The drawing under review shows one solid part. Ordinate dimensions are in mm from its lowest x, y, z. A direction names the side the tool comes from. Coordinates: 2 decimals unless noted, no trailing zeros. Order: outer loops, then holes, each group sorted by start corner. A loop starts at its lowest first (then second) coordinate and runs counter-clockwise, first axis right, second up. Notation, with made-up numbers: (80, 74) -> (102, 74) arc R19 ccw to (102, 86) -> close; hole circle Ø10 at (-21.5, 77.5). An arc over 180 degrees is marked (long way). Put each result on its own line as item: value.
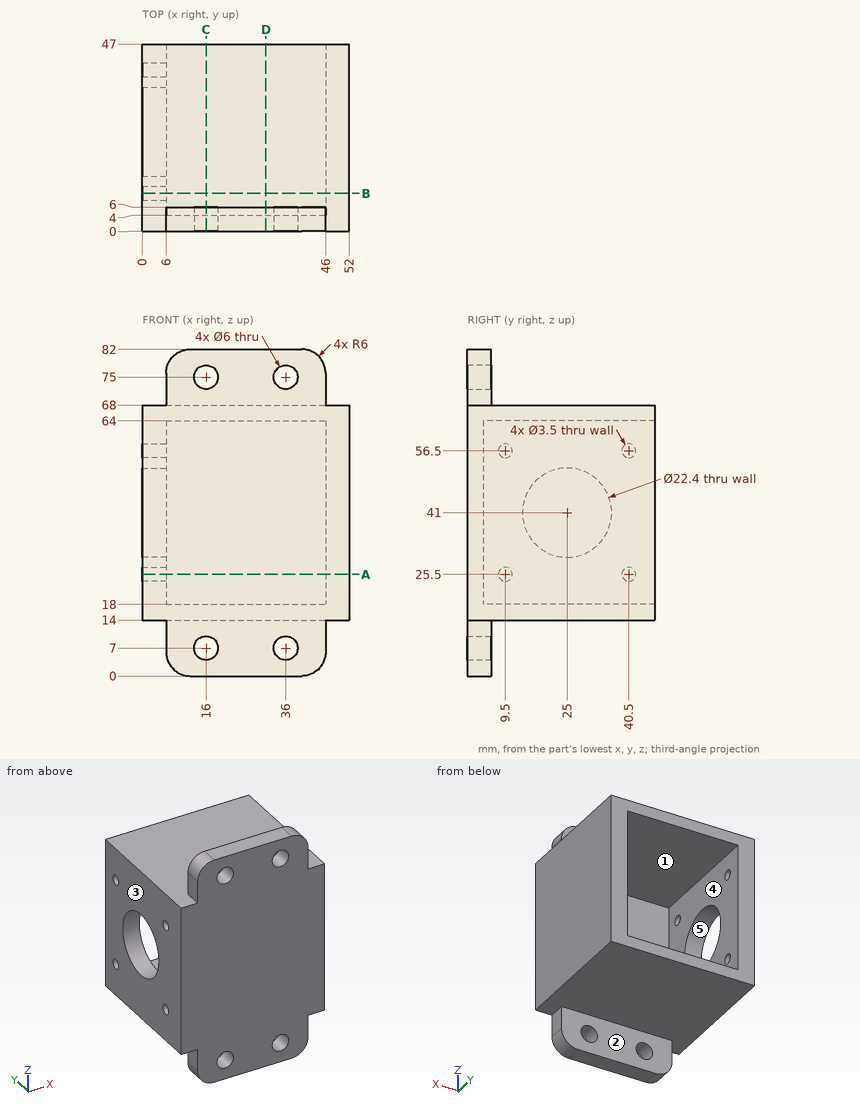
Item 1: Mouldability with a two-part tool opening along Z and no side actions: class the marked faces 1 and 2 as +Z half, -Z half, draft (parallel to the pull), parting line (faces both ways), or undercut.
Answers below:
face 1: undercut
face 2: draft
Item 2: For line 1 (X direction, y = 1, z = 7); line 2 (Y direction, x = 2.7, z = 25.5); line 3 (Z direction, x = 17.5, y = 27.5), list the stretches that pass through material, from the lowest coordinate up. Write a range as from..to.
Answers below:
line 1: 6..13, 19..33, 39..46
line 2: 0..7.75, 11.25..38.75, 42.25..47
line 3: 14..18, 64..68
Item 3: For pin 1 Ø1.8 at (y, z) = (3, 11) entering from -X; pin 2 Ø6 at (x, z) = (33, 10) entering from +Y; pin 3 Ø1.5 at (x, y) = (15, 39.5) entering from -Z, all flat-tipped, find the tip position at first contact; note any pin that passes through.
Answers below:
pin 1: x = 6
pin 2: y = 6
pin 3: z = 14
Item 4: Consider section D-D on x = 31. Write out the cut boundary in (y, z).
Answers below:
outline: (0, 0) -> (6, 0) -> (6, 14) -> (47, 14) -> (47, 18) -> (4, 18) -> (4, 64) -> (47, 64) -> (47, 68) -> (6, 68) -> (6, 82) -> (0, 82) -> close
Item 5: Consider section C-C on x = 16. Write out the cut boundary in (y, z).
Answers below:
outline: (0, 0) -> (6, 0) -> (6, 4) -> (0, 4) -> close; (0, 10) -> (6, 10) -> (6, 14) -> (47, 14) -> (47, 18) -> (4, 18) -> (4, 64) -> (47, 64) -> (47, 68) -> (6, 68) -> (6, 72) -> (0, 72) -> close; (0, 78) -> (6, 78) -> (6, 82) -> (0, 82) -> close
Item 6: For the marked faces 3, 4 and 5, list the 3-axis set-ups (+Z, -Z, +X, -X, +Y, -Y) from which the entire face can be reached by the end or side of a thin tool; tool diameter is ignored.
Answers below:
face 3: +Z, -Z, -X, +Y, -Y
face 4: +Y
face 5: -X
Item 7: Consider section A-A on z = 25.5. Write out the cut boundary in (x, y).
Answers below:
outline: (0, 0) -> (52, 0) -> (52, 47) -> (46, 47) -> (46, 4) -> (6, 4) -> (6, 7.75) -> (0, 7.75) -> close; (0, 11.25) -> (6, 11.25) -> (6, 38.75) -> (0, 38.75) -> close; (0, 42.25) -> (6, 42.25) -> (6, 47) -> (0, 47) -> close
Item 8: Consider section B-B on y = 9.5. Write out the cut boundary in (x, z).
Answers below:
outline: (0, 14) -> (52, 14) -> (52, 68) -> (0, 68) -> (0, 58.25) -> (6, 58.25) -> (6, 64) -> (46, 64) -> (46, 18) -> (6, 18) -> (6, 23.75) -> (0, 23.75) -> close; (0, 27.25) -> (6, 27.25) -> (6, 54.75) -> (0, 54.75) -> close
